Part print with two shaded views. Sizes in mm from the minimum x, y, z corner. A direction names the side the tool comes from. Coordinates: 2 decimals unless noted, no trailing zeros. Loops run counter-clockwise (first coordinate to the right, second up) from the corner with the lowest first, then second, coordinate; pieces in that order, holes last.
(1) Slice it at C-C (z = 5.5). Give the cut face in (x, y).
(2) Slice it at B-B (y = 4). Give the cut face in (x, z), and give its area (4 significant figures).
(3) Slice it at A-A (x = 36). Give the cut face in (y, z).
(4) Tool access for the marked faces 1, 2 and 3: list every direction of +Z, -Z, +X, -X, +Y, -Y with a clear straight run to the whole face (end or side of a thin tool).
(5) Flat gauge pins, fed straight in: P1, Ø1.2, axis at y = 3.5, z = 0.5, coming from the -X side; P2, Ø2.5, axis at x = 24, y = 3.5, coming from the +Z side. Where does each tip first touch, or does it go through?
(6) Two-plate mould, pull along Y, no slides. Class the marked faces 4, 5 and 6: pulls with the +Y half, pulls with the -Y half, needs draft (parallel to the pull), parting line crosses it, or undercut.
(7) Slice it at D-D (y = 2). Give the cut face in (x, z), and give its area (4 significant figures).
(8) Wall check: L1, parallel to X at y = 1.5, z = 5.25; L2, parallel to X at y = 3.5, z = 7.75; L3, parallel to Y at x = 18, z = 3.5. Give the ranges that are in metal, low to high.
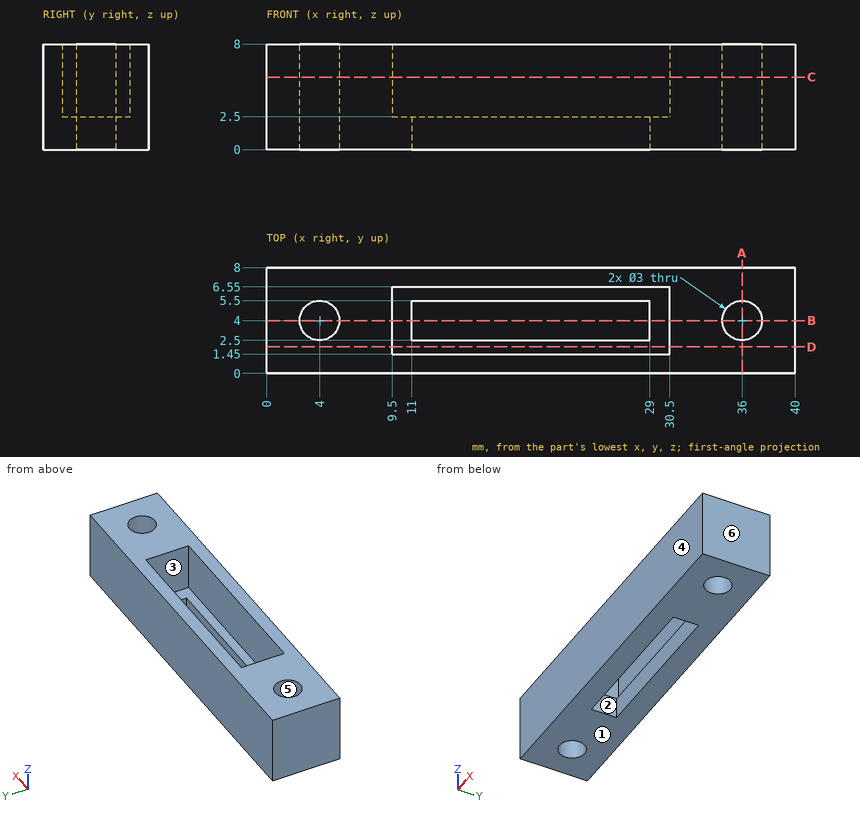
Response values:
1. outline: (0, 0) - (40, 0) - (40, 8) - (0, 8) - close; hole circle Ø3 at (4, 4); hole (9.5, 1.45) - (30.5, 1.45) - (30.5, 6.55) - (9.5, 6.55) - close; hole circle Ø3 at (36, 4)
2. outline: (0, 0) - (2.5, 0) - (2.5, 8) - (0, 8) - close; (5.5, 0) - (11, 0) - (11, 2.5) - (9.5, 2.5) - (9.5, 8) - (5.5, 8) - close; (29, 0) - (34.5, 0) - (34.5, 8) - (30.5, 8) - (30.5, 2.5) - (29, 2.5) - close; (37.5, 0) - (40, 0) - (40, 8) - (37.5, 8) - close
2. area: 111.5 mm2
3. outline: (0, 0) - (2.5, 0) - (2.5, 8) - (0, 8) - close; (5.5, 0) - (8, 0) - (8, 8) - (5.5, 8) - close
4. face 1: -Z, +X, -X, +Y, -Y
4. face 2: +Z, -Z
4. face 3: +Z
5. P1: stops at x = 0
5. P2: stops at z = 2.5
6. face 4: pulls with the -Y half
6. face 5: undercut
6. face 6: needs draft
7. outline: (0, 0) - (40, 0) - (40, 8) - (30.5, 8) - (30.5, 2.5) - (9.5, 2.5) - (9.5, 8) - (0, 8) - close
7. area: 204.5 mm2
8. L1: x = 0 to 9.5, 30.5 to 40
8. L2: x = 0 to 2.59, 5.41 to 9.5, 30.5 to 34.59, 37.41 to 40
8. L3: y = 0 to 1.45, 6.55 to 8
